Solid Edge part; units mm, degrees
sketch "Sketch1" plane through (0, 0, 0) normal (0, -1, 0) x (1, 0, 0)
  line L0 (5.7735, 10) -> (-5.7735, 10)
  line L1 (-5.7735, 10) -> (-11.547, 0)
  line L2 (-11.547, 0) -> (-5.7735, -10)
  line L3 (-5.7735, -10) -> (5.7735, -10)
  line L4 (5.7735, -10) -> (11.547, 0)
  line L5 (11.547, 0) -> (5.7735, 10)
  circle A0 centre (0, 0) radius 5
extrude "Protrusion1" add sketch "Sketch1" along normal mid plane 5
Build history of the part. All positions in model axes, mm. Give positions to 0.01 mm unless a question says otherwise; leave off trailing zeros. Order: outer loops, then holes, each group sorted by start corner. A loop starts at its lowest first (then second) coordinate and runs counter-clockwise, first axis right, second up. Notation, with made-up numbers: M 57.25,66 L 105.25,66 A5 cw 105.25,70 Z; hole C -37.75,9.25 d3. An arc over 180 degrees is marked long. Return JSON: item names as keys, results as strings.
Q1. Band-saw the part on B-B (y = -1.05). Give the cut face in (x, z).
Answer list:
{"outline": "M -11.55,0 L -5.77,-10 L 5.77,-10 L 11.55,0 L 5.77,10 L -5.77,10 Z; hole C 0,0 d10"}
Q2. Band-saw the part on A-A (x = 0). Give the cut face in (y, z).
Answer list:
{"outline": "M -2.5,-10 L 2.5,-10 L 2.5,-5 L -2.5,-5 Z; M -2.5,5 L 2.5,5 L 2.5,10 L -2.5,10 Z"}
Q3. Band-saw the part on C-C (z = -3). Give the cut face in (x, y).
Answer list:
{"outline": "M -9.81,-2.5 L -4,-2.5 L -4,2.5 L -9.81,2.5 Z; M 4,-2.5 L 9.81,-2.5 L 9.81,2.5 L 4,2.5 Z"}
Q4. Flat gauge pins, fed straight in: pin 1 (1 mm diameter, centred on x = 7, y = 1, fed in from -Z); pin 2 (1 mm diameter, centred on x = -8, y = -1.5, fed in from +Z); pin 3 (1 mm diameter, centred on y = -0.5, z = 7.5, fed in from -X). Where does each tip first touch, or does it go through?
Answer list:
{"pin 1": "stops at z = -8.74", "pin 2": "stops at z = 7.01", "pin 3": "stops at x = -7.51"}
Q5. Band-saw the part on D-D (x = 7.5). Give the cut face in (y, z), then the cut area to 3 significant figures.
Answer list:
{"outline": "M -2.5,-7.01 L 2.5,-7.01 L 2.5,7.01 L -2.5,7.01 Z", "area": "70.1 mm^2"}
Q6. Wall check: probe 1 along Z at (x, y) = (0, 0.9); probe 2 along Z at (x, y) = (1, 1.05); probe 3 along Z at (x, y) = (-7.25, -0.5). Give the ranges that are in metal, low to high. Write a range as from..to.
Answer list:
{"probe 1": "z = -10..-5, 5..10", "probe 2": "z = -10..-4.9, 4.9..10", "probe 3": "z = -7.44..7.44"}
Q7. Two-plate mould, pull along Z, no slides. Class faces 1 (the face through (-1.08, 0.04, 4.88)), 2 (the face through (-2, -2.5, 5)), 3 (the face through (-8.62, 0.04, 5.07)): pulls with the +Z half, pulls with the -Z half, needs draft (parallel to the pull), parting line crosses it, or undercut.
Answer list:
{"face 1": "undercut", "face 2": "needs draft", "face 3": "pulls with the +Z half"}
